```python
from build123d import *

# Parameters (mm, degrees)
F0_W     = 50.8
F0_H     = 152.4
F0_R     = 2.032
F0_R_2   = 13.97
F1_DEPTH = 5.334
F2_R     = 3.175
F3_DEPTH = 25.4


with BuildPart() as f1:
    # F0 (on Top) → F1 (new body)
    with BuildSketch(Plane.XY):
        with Locations((-18.054181, 9.979866)):
            Rectangle(F0_W, F0_H)
        with Locations((-36.011981, -3.240235)):
            Circle(F0_R, mode=Mode.SUBTRACT)
        with Locations((-18.054181, -2.720134)):
            Circle(F0_R_2, mode=Mode.SUBTRACT)
        with Locations((-17.53408, -20.677934)):
            Circle(F0_R, mode=Mode.SUBTRACT)
        with Locations((-0.096381, -2.200033)):
            Circle(F0_R, mode=Mode.SUBTRACT)
        with Locations((-18.574282, 15.237666)):
            Circle(F0_R, mode=Mode.SUBTRACT)
        with Locations((-18.377712, 42.822066)):
            Circle(F0_R, mode=Mode.SUBTRACT)
        with Locations((-36.011981, 61.103397)):
            Circle(F0_R, mode=Mode.SUBTRACT)
        with Locations((-18.054181, 60.779866)):
            Circle(F0_R_2, mode=Mode.SUBTRACT)
        with Locations((-17.730651, 78.737666)):
            Circle(F0_R, mode=Mode.SUBTRACT)
        with Locations((-0.096381, 60.456336)):
            Circle(F0_R, mode=Mode.SUBTRACT)
    extrude(amount=F1_DEPTH)

    # F2 (on face) → F3 (cut)
    with BuildSketch(Plane(origin=(0, 0, 0), x_dir=(1, 0, 0), z_dir=(0, 0, -1))):
        with Locations((-5.354181, 48.440134)):
            Circle(F2_R)
        with Locations((-30.754181, 48.440134)):
            Circle(F2_R)
    extrude(amount=-F3_DEPTH, mode=Mode.SUBTRACT)


solid = f1.part
```
Input: part model. Units: mm. Frame: model coordinates. Coordinates: 2 decimals unless noted, no trailing zeros. Loops run counter-clockwise (first coordinate to the right, second up) from the corner with the lowest first, then second, coordinate; pieces in that order, holes last. Notation, with made-up numbers: M -23,64.5 L 35,64.5 A33 ccw 35,98.5 Z; hole C -2,30 d10. An arc over 180 degrees is marked long. Use a Markdown table: item, result. Add a question column.
1) Section B-B, the plane x = -0.5. Return the cut outline in (y, z), plus the area to 3 significant figures.
2) Section A-A, the plane y = 4. Return the cut outline in (x, z).
3) Section C-C, the plane z = 3.8. Give the number of separate pieces and of enclosed holes in the cut face, plus the area to 3 significant figures.
4) Section D-D, the plane y = 68. Return the cut outline in (x, z), plus the area to 3 significant figures.
5) Draft query along X for faces 1 (the flat face through (-18, -66.22, 3)), 2 (the cylindrical face through (-20.187, 14.001, 2.63)), 3 (the flat face through (7.346, 9, 3)). Return one class per face: +X half, -X half, draft (parallel to the pull), parting line (faces both ways), or undercut.
6) Line query: L1, parallel to Y at x = -13, z = 1.2; L2, parallel to Y at x = -27, z = 2.85; L3, parallel to Y at x = -28.5, z = 0.65. Output: solid intervals per line, ascending. Write a range as from..to.
Answer below:
| question | item | result |
|---|---|---|
| 1 | outline | M -66.22,0 L -4.19,0 L -4.19,5.33 L -66.22,5.33 Z; M -0.21,0 L 58.46,0 L 58.46,5.33 L -0.21,5.33 Z; M 62.45,0 L 86.18,0 L 86.18,5.33 L 62.45,5.33 Z |
| 1 | area | 770 mm2 |
| 2 | outline | M -43.45,0 L -30.3,0 L -30.3,5.33 L -43.45,5.33 Z; M -5.81,0 L 7.35,0 L 7.35,5.33 L -5.81,5.33 Z |
| 3 | separate pieces | 1 |
| 3 | enclosed holes | 12 |
| 3 | area | 6,350 mm2 |
| 4 | outline | M -43.45,0 L -30.01,0 L -30.01,5.33 L -43.45,5.33 Z; M -6.09,0 L 7.35,0 L 7.35,5.33 L -6.09,5.33 Z |
| 4 | area | 143 mm2 |
| 5 | face 1 | draft |
| 5 | face 2 | undercut |
| 5 | face 3 | +X half |
| 6 | L1 | -66.22..-15.74, 10.3..47.76, 73.8..86.18 |
| 6 | L2 | -66.22..-13.45, 8.01..50.05, 71.51..86.18 |
| 6 | L3 | -66.22..-50.68, -46.2..-12, 6.56..51.5, 70.06..86.18 |
